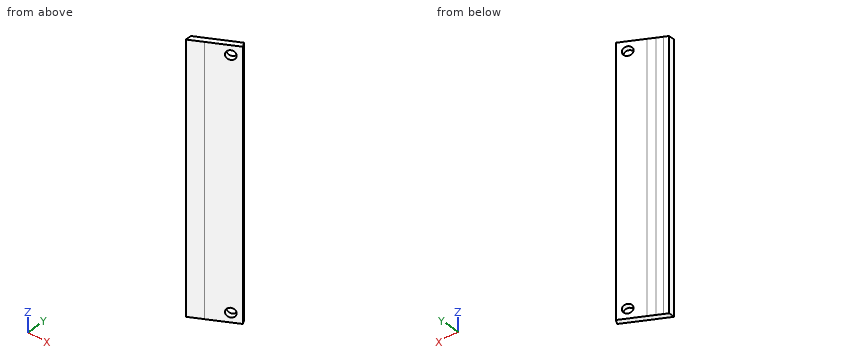
Autodesk Inventor part; units mm, degrees
ref_plane "YZ Plane" through (0, 0, 0) normal (1, 0, 0) x (0, 1, 0)
ref_plane "XZ Plane" through (0, 0, 0) normal (0, 1, 0) x (-1, 0, 0)
ref_plane "XY Plane" through (0, 0, 0) normal (0, 0, 1) x (1, 0, 0)
sketch "Szkic1" plane through (0, 0, 0) normal (0, 0, 1) x (1, 0, 0)
  line L0 (0, 0) -> (0, -66.5)
  line L1 (0, -66.5) -> (2, -66.5)
  line L2 (2, 0) -> (2, -66.5)
  line L3 (0, 0) -> (2, 0)
  circle A0 centre (7, 15.8) radius 1.5
  circle A1 centre (7, 15.8) radius 15.02
  line L4 (7, 30.82) -> (7, 14.3)
  line L5 (7, -69.18) -> (-7.0129, -69.18)
  line L6 (37, -46.3508) -> (4.3309, -63.8229)
  line L7 (37, -48.6189) -> (3.5105, -66.5297)
  line L8 (37, -48.6189) -> (37, -46.3508)
  line L9 (37, -48.6189) -> (-1.4451, -69.18)
  line L10 (37, -46.3508) -> (-1.4451, -66.9119)
  line L11 (-1.4451, -66.9119) -> (-1.4451, -69.18)
  dimension "d0" = 100
extrude "Wyciągnięcie proste1" add sketch "Szkic1" against normal blind 100 contours L10 L2 L1 L0 | L0 L1 L2 L10 L6 L8 L7 L9 L11
sketch "Szkic5" plane through (-1.4451, -69.18, -100) normal (0.4716, -0.8818, 0) x (0.8818, 0.4716, 0)
  line L0 (17.9345, 9.0111) -> (17.7164, 38.6148)
  line L1 (17.7164, 38.6148) -> (26.2335, 38.9662)
  line L2 (26.4517, 9.3625) -> (17.9345, 9.0111)
  line L3 (26.2335, 38.9662) -> (17.9345, 38.9662)
  line L4 (17.9345, 38.9662) -> (17.9345, 9.0111)
  line L5 (17.9345, 9.0111) -> (26.2335, 9.0111)
  line L6 (26.2335, 9.0111) -> (26.2335, 38.9662)
  line L7 (17.4345, 39.4662) -> (26.7335, 39.4662)
  line L8 (26.7335, 39.4662) -> (26.7335, 8.5111)
  line L9 (26.7335, 8.5111) -> (17.4345, 8.5111)
  line L10 (17.4345, 8.5111) -> (17.4345, 39.4662)
  line L11 (17.4345, 39.4662) -> (16.9345, 39.4662)
  line L12 (16.9345, 39.4662) -> (16.9345, 8.5111)
  line L13 (16.9345, 8.5111) -> (17.4345, 8.5111)
  line L14 (17.4345, 8.5111) -> (17.4345, 39.4662)
  line L15 (26.7335, 38.9662) -> (16.9345, 38.9662)
  line L16 (16.9345, 38.9662) -> (16.9345, 9.0111)
  line L17 (16.9345, 9.0111) -> (26.7335, 9.0111)
  line L18 (26.7335, 9.0111) -> (26.7335, 38.9662)
  point P0 (33.9001, 100)
  point P1 (17.9345, 9.0111)
  point P2 (26.7335, 9.0111)
  point P3 (17.9345, 38.9662)
  dimension "d7" = 0.5
  dimension "d8" = 0.5
extrude "Wyciągnięcie proste4" cut sketch "Szkic5" against normal through all contours L17 L10 L15 L4 L1 L0 | L4 L1 L6 L2 | L0 L1 L4 | L2 L6 L5 | L6 L15 L8 L17 | L4 L3 L1 | L17 L12 L15 L10
ref_plane "Płaszczyzna konstrukcyjna1" through (0, 0, -50) normal (0, 0, 1) x (1, 0, 0)
mirror "Odbij1" about plane through (0, 0, -50) normal (0, 0, 1) of "Wyciągnięcie proste4"
sketch "Szkic6" plane through (-1.4451, -69.18, -100) normal (0.4716, -0.8818, 0) x (0.8818, 0.4716, 0)
  line L0 (16.9345, 61.0338) -> (16.9345, 38.9662)
  line L1 (44.6676, 100) -> (16.9345, 100)
  line L2 (44.6676, 100) -> (44.6676, 0)
  line L3 (16.9345, 0) -> (44.6676, 0)
  line L4 (16.9345, 9.0111) -> (26.7335, 9.0111)
  line L5 (26.7335, 9.0111) -> (26.7335, 38.9662)
  line L6 (26.7335, 38.9662) -> (16.9345, 38.9662)
  line L7 (16.9345, 61.0338) -> (26.7335, 61.0338)
  line L8 (26.7335, 61.0338) -> (26.7335, 90.9889)
  line L9 (26.7335, 90.9889) -> (16.9345, 90.9889)
  circle A0 centre (32.598, 3.55) radius 1.75
  circle A1 centre (32.598, 96.45) radius 1.75
  line L10 (16.9345, 90.9889) -> (16.9345, 100)
  line L11 (16.9345, 0) -> (16.9345, 9.0111)
  line L12 (16.9345, 38.9662) -> (16.9345, 61.0338)
  point P0 (33.9001, 100)
extrude "Wyciągnięcie proste5" [suppressed]
sketch "Szkic7" plane through (-1.4451, -69.18, -100) normal (0.4716, -0.8818, 0) x (0.8818, 0.4716, 0)
  line L0 (0, 100) -> (43.598, 100)
  line L1 (0, 100) -> (0, 0)
  line L2 (43.598, 0) -> (0, 0)
  line L3 (16.9345, 100) -> (0, 100)
  line L4 (0, 100) -> (0, 92.9)
  line L5 (0, 92.9) -> (16.9345, 92.9)
  line L6 (16.9345, 92.9) -> (16.9345, 100)
  circle A0 centre (13.3845, 96.45) radius 3.55
  circle A1 centre (13.3845, 96.45) radius 1.75
  line L7 (-8.9335, 50) -> (53.6011, 50)
  circle A2 centre (13.3845, 3.55) radius 1.75
  line L8 (43.598, 100) -> (43.598, 0)
  point P0 (33.9001, 100)
  dimension "d13" = 7.1
  dimension "d14" = 3.5
extrude "Wyciągnięcie proste6" cut sketch "Szkic7" against normal through all contours A1 | A2
sketch "Szkic8" plane through (-1.4451, -69.18, -100) normal (0.4716, -0.8818, 0) x (0.8818, 0.4716, 0)
  circle A0 centre (13.3845, 3.55) radius 1.75
  circle A1 centre (13.3845, 96.45) radius 1.75
  line L0 (16.9345, 61.0338) -> (16.9345, 90.9889)
  line L1 (16.9345, 90.9889) -> (26.7335, 90.9889)
  line L2 (26.7335, 90.9889) -> (26.7335, 61.0338)
  line L3 (26.7335, 61.0338) -> (16.9345, 61.0338)
  line L4 (26.7335, 38.9662) -> (26.7335, 9.0111)
  line L5 (26.7335, 9.0111) -> (16.9345, 9.0111)
  line L6 (16.9345, 9.0111) -> (16.9345, 38.9662)
  line L7 (16.9345, 38.9662) -> (26.7335, 38.9662)
  line L8 (0, 100) -> (43.598, 100)
  line L9 (0, 100) -> (0, 0)
  line L10 (43.598, 0) -> (0, 0)
  line L11 (43.598, 100) -> (43.598, 0)
  line L12 (43.598, 100) -> (44.6676, 100)
  line L13 (43.598, 100) -> (43.598, 0)
  line L14 (44.6676, 0) -> (43.598, 0)
  line L15 (44.6676, 100) -> (44.6676, 0)
  line L16 (44.6676, 100) -> (16.9345, 100)
  line L17 (16.9345, 100) -> (16.9345, 0)
  line L18 (16.9345, 0) -> (44.6676, 0)
  line L19 (44.6676, 0) -> (44.6676, 100)
  point P0 (33.9001, 100)
  point P1 (16.9345, 61.0338)
  point P2 (16.9345, 38.9662)
  point P3 (16.9345, 9.0111)
  point P4 (16.9345, 100)
  point P5 (16.9345, 90.9889)
extrude "Wyciągnięcie proste7" cut sketch "Szkic8" against normal through all contours L3 L2 L1 L17 L8 L11 L10 L5 L4 L7 | L12 L15 L14 L11
properties part number "plug_kopia"
Model file for the job. Use its own axes, mm. Round coordinates to 2 decimals unless told otherwise and drop trailing zeros. Loops run counter-clockwise (first coordinate to the right, second up) from the corner with the lowest first, then second, coordinate; pieces in that order, holes last. Notation, with made-up numbers: (37, 21) -> (61, 21) arc R24 cw to (61, 47) -> close; hole circle Ø2 at (-26.5, 62.5). An arc over 180 degrees is marked (long way). Answer as CSV lines item,"result". Start each with the question number.
1) Probe line 1 along Y through (x, z) = (10.25, -67); line 2 along Y through (x, z) = (6.25, -52.5); line 3 along X through (y, z) = (-68, -73.5). List the from-to ranges inside material, lowest first.
2) Pin check, flat tips, straight feed: P1, Ø5, axis at y = -66, z = -51.5, coming from the -X side; P2, Ø1, axis at x = 0, z = -50, coming from the +Y side; P3, Ø3, axis at x = 2.5, z = -65, coming from the -Y side; P4, Ø1.5, axis at x = 1.5, z = -76, coming from the -Y side. Stop position of each tip, or through.
3) Slice it at B-B (x = 9). State how many separate pieces and enclosed holes the cut face has, plus the area to 3 significant figures.
4) Slice it at A-A (z = -64.5). List the corners of the cut face in (x, y), plus the area to 3 significant figures.
5) Slice it at C-C (x = 5.25). List the corners of the cut face in (y, z), plus the area to 3 significant figures.
Filled in:
1,line 1,"y = -62.93 to -60.66"
1,line 2,"y = -65.06 to -62.8"
1,line 3,"x = -1.45 to 0.76"
2,P1,"stops at x = -1.45"
2,P2,"stops at y = -65.87"
2,P3,"stops at y = -67.87"
2,P4,"stops at y = -68.01"
3,separate pieces,"3"
3,enclosed holes,"0"
3,area,"214 mm2"
4,outline,"(-1.45, -69.18) -> (3.51, -66.53) -> (13.49, -61.19) -> (12.54, -59.43) -> (4.33, -63.82) -> (-1.45, -66.91) -> close"
4,area,"32.8 mm2"
5,outline,"(-65.6, -100) -> (-63.33, -100) -> (-63.33, 0) -> (-65.6, 0) -> close"
5,area,"227 mm2"
